Here's the drawing with two shaded views (mm, measured from the low corner). I have some questions. A direction names the side the tool comes from. Give positions to 0.01 mm unless a question says otherwise; leave off trailing zeros. Loops run counter-clockwise (first coordinate to the right, second up) from the corner with the lowest first, then second, coordinate; pieces in that order, holes last.
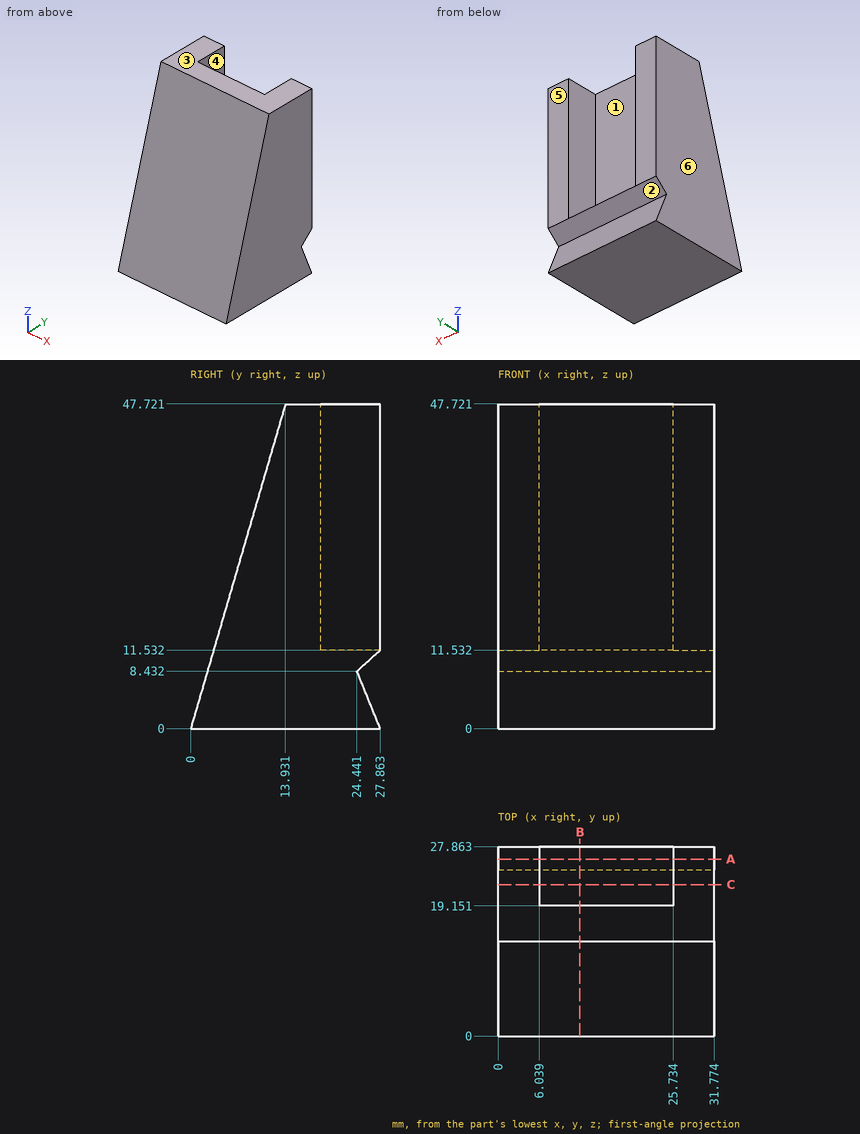
(1) Will these pins go through, and if not, where does the flat tip stop? P1, Ø5, axis at x = 16.5, z = 38, coming from the -Y side; P2, Ø2, axis at y = 7, z = 34.5, coming from the +X side; P3, Ø2, axis at x = 21.5, z = 25, coming from the -Y side; P4, Ø1, axis at x = 19, z = 24, coming from the -Y side.
Returned:
P1: stops at y = 10.36
P2: passes through
P3: stops at y = 7.01
P4: stops at y = 6.86
(2) Suppose I cut it at A-A on y = 26. List the corners of the cut face in (x, z) for me (1 decimal).
Returned:
outline: (0, 0) - (31.8, 0) - (31.8, 4.6) - (0, 4.6) - close; (0, 9.8) - (31.8, 9.8) - (31.8, 47.7) - (25.7, 47.7) - (25.7, 11.5) - (6, 11.5) - (6, 47.7) - (0, 47.7) - close
(3) Suppose I cut it at C-C on y = 22.25. List the corners of the cut face in (x, z) for me (1 decimal).
Returned:
outline: (0, 0) - (31.8, 0) - (31.8, 47.7) - (25.7, 47.7) - (25.7, 11.5) - (6, 11.5) - (6, 47.7) - (0, 47.7) - close
(4) Thinking about a two-plate mould opening in X: for the marked faces 4, 5 and 6, which applies, pulls with the +X half, pulls with the -X half, needs draft (parallel to the pull), parting line crosses it, or undercut?
Returned:
face 4: undercut
face 5: needs draft
face 6: pulls with the -X half
(5) Which directions (+Z, -Z, +X, -X, +Y, -Y) give clear straight access to the entire face, cutting with the end or side of a thin tool? Please do the marked faces 1, 2 and 3.
Returned:
face 1: +Z, +Y
face 2: +X, -X, +Y
face 3: +Z, +X, -X, +Y, -Y
(6) Suppose I cut it at B-B on x = 12. List the corners of the cut face in (y, z) for me, plus the area to 3 significant figures.
Returned:
outline: (0, 0) - (27.86, 0) - (24.44, 8.43) - (27.86, 11.53) - (19.15, 11.53) - (19.15, 47.72) - (13.93, 47.72) - close
area: 662 mm2
(7) Please list where these lines run through material, in increasing order: probe 1 along X at (y, z) = (24.25, 33) (1 decimal); probe 2 along Z at (x, y) = (7.5, 24.75) (1 decimal); probe 3 along Y at (x, z) = (21, 12).
Returned:
probe 1: x = 0 to 6, 25.7 to 31.8
probe 2: z = 0 to 7.7, 8.7 to 11.5
probe 3: y = 3.5 to 19.15
